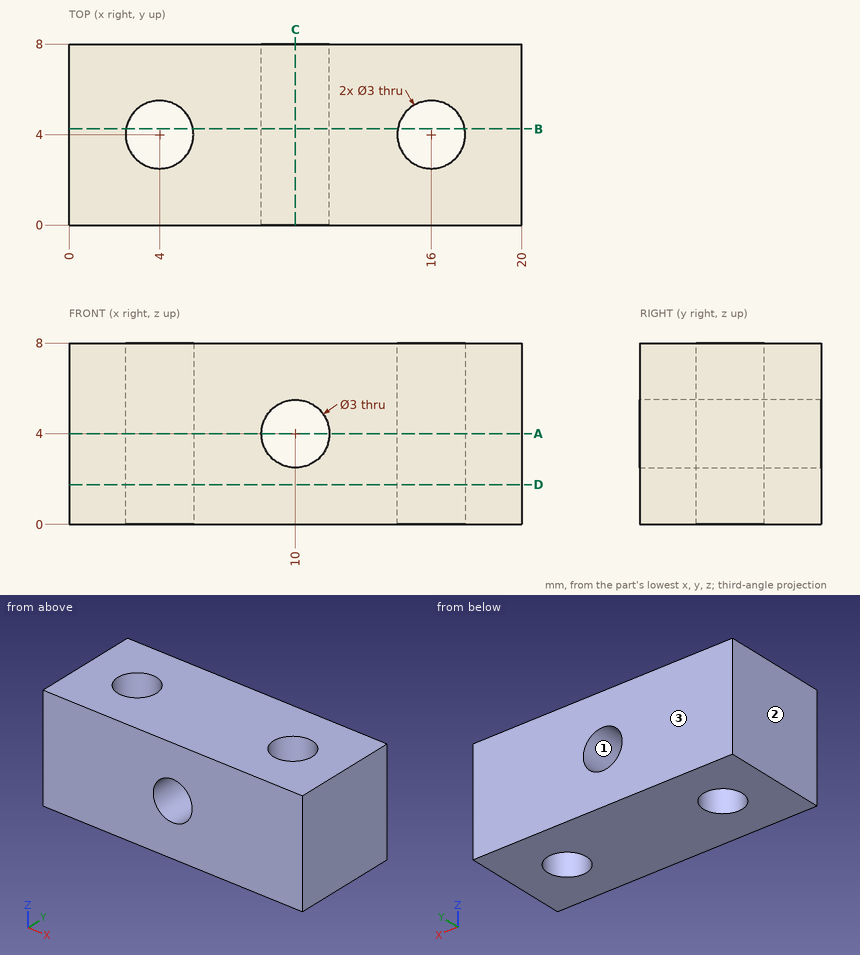
The figure shows three views and two pictorial views of one solid part (mm, origin at its lowest corner). Answer the questions. Give positions to 0.01 mm unless a question says otherwise; leave off trailing zeros. Order: outer loops, then holes, each group sorted by start corner. A loop starts at its lowest first (then second) coordinate and runs counter-clockwise, first axis right, second up. Notation, with made-up numbers: M 36.25,-32 L 88.25,-32 A14 cw 88.25,-16 Z; hole C -26.75,51.25 d9. An arc over 180 degrees is marked long. Return JSON: item names as keys, results as strings.
Q1. Find section B-B, the plane y = 4.25. Write down the section's boundary in (x, z), and give its area (3 significant figures).
Answer below:
{"outline": "M 0,0 L 2.52,0 L 2.52,8 L 0,8 Z; M 5.48,0 L 14.52,0 L 14.52,8 L 5.48,8 Z; M 17.48,0 L 20,0 L 20,8 L 17.48,8 Z; hole C 10,4 d3", "area": "106 mm^2"}
Q2. Find section C-C, the plane x = 10. Write down the section's boundary in (y, z).
Answer below:
{"outline": "M 0,0 L 8,0 L 8,2.5 L 0,2.5 Z; M 0,5.5 L 8,5.5 L 8,8 L 0,8 Z"}
Q3. Find section A-A, the plane z = 4. Write down the section's boundary in (x, y), and give its area (3 significant figures).
Answer below:
{"outline": "M 0,0 L 8.5,0 L 8.5,8 L 0,8 Z; M 11.5,0 L 20,0 L 20,8 L 11.5,8 Z; hole C 4,4 d3; hole C 16,4 d3", "area": "122 mm^2"}
Q4. Find section D-D, the plane z = 1.75. Write down the section's boundary in (x, y).
Answer below:
{"outline": "M 0,0 L 20,0 L 20,8 L 0,8 Z; hole C 4,4 d3; hole C 16,4 d3"}
Q5. The mould has two halves that part along X. Classify the marked faces 1, 2 and 3: pulls with the +X half, pulls with the -X half, needs draft (parallel to the pull), parting line crosses it, or undercut.
Answer below:
{"face 1": "undercut", "face 2": "pulls with the -X half", "face 3": "needs draft"}
Q6. Find the intervals of material crossed by line 1 along Y through (x, z) = (4, 6.5); line 2 along X through (y, z) = (2, 4); line 3 along X through (y, z) = (3.5, 7.5), in increasing order. Write a range as [from, to].
Answer below:
{"line 1": "y = [0, 2.5], [5.5, 8]", "line 2": "x = [0, 8.5], [11.5, 20]", "line 3": "x = [0, 2.59], [5.41, 14.59], [17.41, 20]"}
